from build123d import *

# Parameters (mm, degrees)
BOSS_EXTRUDE1_DEPTH     = 50
BOSS_EXTRUDE2_DEPTH     = 10
BOSS_EXTRUDE3_START     = 30
BOSS_EXTRUDE3_DEPTH     = 10
SKETCH3_W               = 12
SKETCH3_H               = 10
BOSS_EXTRUDE4_DEPTH     = 15
CUT_EXTRUDE1_DEPTH      = 119.427192823
CUT_EXTRUDE1_DEPTH_BACK = 119.427192823
SKETCH4_R               = 3
SKETCH4_W               = 28
SKETCH4_H               = 4


with BuildPart() as part:
    # Sketch1 → Boss-Extrude1 (new body)
    with BuildSketch(Plane.XY):
        Polygon((69.618802154, 8), (65, 0), (80, 0), (80, 17.220839506), (0, 17.220839506), (0, 0), (15, 0), (10.381197846, 8), align=None)
    extrude(amount=BOSS_EXTRUDE1_DEPTH)

    # Sketch2 → Boss-Extrude2 (add)
    with BuildSketch(Plane.XY):
        Polygon((0, 17.220839506), (80, 17.220839506), (95, 40.639434385), (95, 50), (-15, 50), (-15, 39.999070977), align=None)
    extrude(amount=BOSS_EXTRUDE2_DEPTH)

    # Sketch2_3 → Boss-Extrude3 (add)
    with BuildSketch(Plane.XY.offset(BOSS_EXTRUDE3_START)):
        Polygon((0, 17.220839506), (80, 17.220839506), (95, 40.639434385), (95, 50), (-15, 50), (-15, 39.999070977), align=None)
    extrude(amount=BOSS_EXTRUDE3_DEPTH)

    # Sketch3 → Boss-Extrude4 (add)
    with BuildSketch(Plane(origin=(0, 17.220839506, 0), x_dir=(1, 0, 0), z_dir=(0, 1, 0))):
        with Locations((51.419853225, -20.126174842)):
            Rectangle(SKETCH3_W, SKETCH3_H)
    extrude(amount=BOSS_EXTRUDE4_DEPTH)

    # Sketch4 → Cut-Extrude1 (cut, two sides: drawn at the far end of the back side and taken through both)
    with BuildSketch(Plane(origin=(0, 0, 0), x_dir=(0, 0, -1), z_dir=(1, 0, 0)).offset(-CUT_EXTRUDE1_DEPTH_BACK)):
        with Locations(Location((-20.126174842, 25.220839506, 0), (0, 0, 180))):
            Circle(SKETCH4_R)
        with Locations((-20, 48)):
            Rectangle(SKETCH4_W, SKETCH4_H)
    extrude(amount=CUT_EXTRUDE1_DEPTH + CUT_EXTRUDE1_DEPTH_BACK, mode=Mode.SUBTRACT)


solid = part.part
Geometry: final body of the model. Coordinates: model frame, mm. A direction names the side the tool comes from. Round coordinates to 2 decimals unless told otherwise and drop trailing zeros. Loops run counter-clockwise (first coordinate to the right, second up) from the corner with the lowest first, then second, coordinate; pieces in that order, holes last. Notation, with made-up numbers: (81.5, 81.5) - (95.5, 81.5) arc R18 cw to (95.5, 99.5) - close; hole circle Ø10 at (48, 73.5). An arc over 180 degrees is marked (long way). Write each question's results on one line, items separated by ' | '. Start each with the question number.
1) Cut plane B-B on x = 7. Return loops of the section in (y, z), then the cut area to 3 significant figures.
2) Cut plane A-A on y = 21. Return loops of the section in (x, z).
3) Cut plane D-D on z = 7.5. Return loops of the section in (x, y), then the cut area to 3 significant figures.
4) Cut plane C-C on z = 21. Return loops of the section in (x, y), then the cut area to 3 significant figures.
5) Mould query, pull axis Y, two halves, no side actions, for faces 1 (the face through (87.395, 28.766, 34.93)), 2 (the face through (67.342, 4.056, 24.65)), 3 (the face through (0, 9, 25)). Classes: released by +Y, released by -Y, zero draft, split by the parting line, or undercut.
6) Access query for faces 4 (the face through (41, 17.221, 45)), 5 (the face through (12.723, 3.944, 24.65)), 6 (the face through (39, 46, 32)). Directions: +Z, -Z, +X, -X, +Y, -Y. A direction counts if a zero-diameter tool reaches every point of the face in a straight line with its end or side. Return the directions, or none.
7) First-contact query: P1, Ø1.5, axis at y = 35, z = 35.5, coming from the -X side; P2, Ø5, axis at x = 60, z = 45, coming from the +Y side; P3, Ø1, axis at y = 27.5, z = 11, coming from the +X side; P4, Ø1.2, axis at x = 48.5, z = 32.5, coming from the +Y side. Flat tips, straight axial feed; report the tip coordinate or a pass-through.
8) Line query: probe 1 along Z at (x, y) = (47.5, 44.5); probe 2 along Z at (x, y) = (47.5, 31.5); probe 3 along Z at (x, y) = (0, 48.5). Output: solid intervals per line, ascending. Write a range as [from, to].
Verdict:
1) outline: (0, 0) - (50, 0) - (50, 6) - (46, 6) - (46, 10) - (17.22, 10) - (17.22, 30) - (46, 30) - (46, 34) - (50, 34) - (50, 40) - (17.22, 40) - (17.22, 50) - (0, 50) - close | area: 1,480 mm2
2) outline: (-2.49, 0) - (82.42, 0) - (82.42, 10) - (-2.49, 10) - close; (-2.49, 30) - (82.42, 30) - (82.42, 40) - (-2.49, 40) - close; (45.42, 15.13) - (57.42, 15.13) - (57.42, 25.13) - (45.42, 25.13) - close
3) outline: (-15, 40) - (0, 17.22) - (0, 0) - (15, 0) - (10.38, 8) - (69.62, 8) - (65, 0) - (80, 0) - (80, 17.22) - (95, 40.64) - (95, 46) - (-15, 46) - close | area: 3,760 mm2
4) outline: (0, 0) - (15, 0) - (10.38, 8) - (69.62, 8) - (65, 0) - (80, 0) - (80, 17.22) - (57.42, 17.22) - (57.42, 22.35) - (45.42, 22.35) - (45.42, 17.22) - (0, 17.22) - close; (45.42, 28.09) - (57.42, 28.09) - (57.42, 32.22) - (45.42, 32.22) - close | area: 1,050 mm2
5) face 1: released by -Y | face 2: undercut | face 3: zero draft
6) face 4: +Z, +X, -X, +Y | face 5: +Z, -Z | face 6: +X, -X, +Y
7) P1: stops at x = -12.2 | P2: stops at y = 17.22 | P3: passes through | P4: stops at y = 46
8) probe 1: z = [0, 10], [30, 40] | probe 2: z = [0, 10], [15.13, 25.13], [30, 40] | probe 3: z = [0, 6], [34, 40]
